Drawing for the job (mm, zero at the part's lowest x, y, z). A direction names the side the tool comes from. Round coordinates to 2 decimals unless told otherwise and drop trailing zeros. Loops run counter-clockwise (first coordinate to the right, second up) from the corner with the lowest first, then second, coordinate; pieces in that order, holes last. Notation, with made-up numbers: M 34,47.5 L 54,47.5 A21 ccw 54,75.5 Z; hole C 89,32.5 d1. An arc over 180 degrees is marked long. Answer in a Markdown table with one row per item.
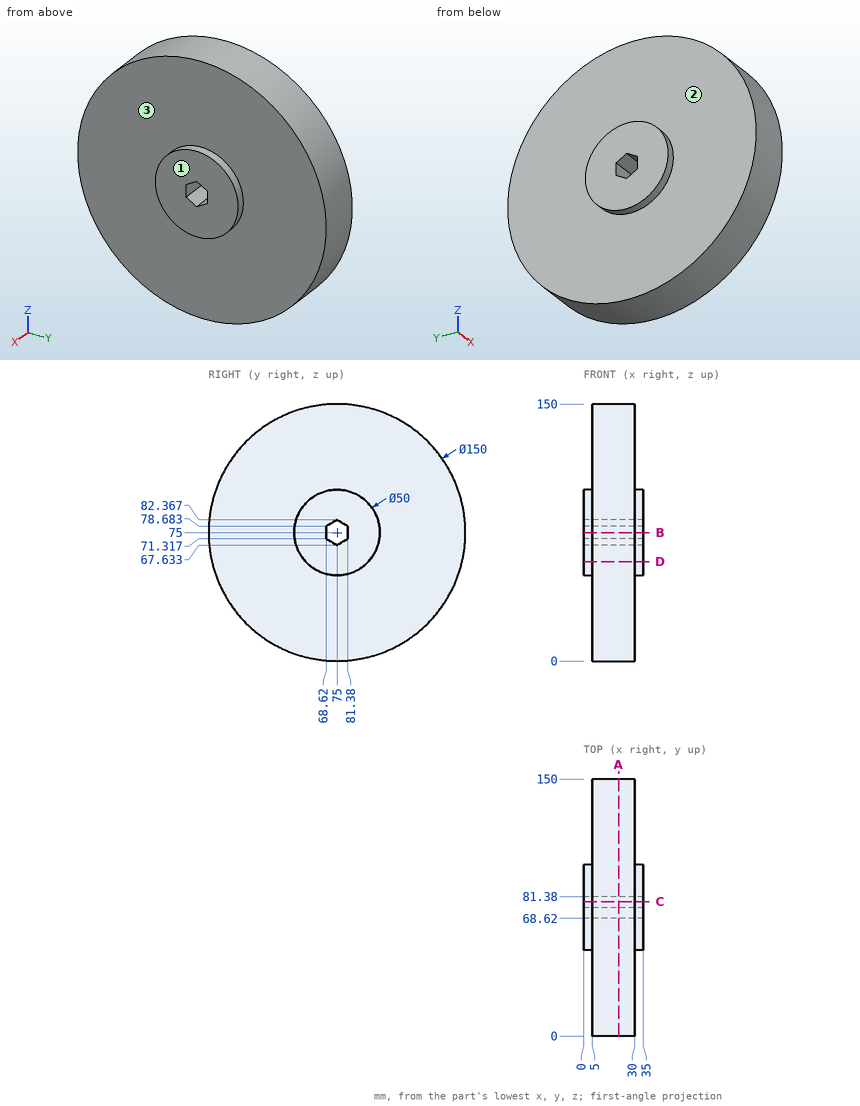
1. Saw through at C-C (y = 78.5). Write the cut outline in (x, z).
Verdict:
| item | result |
|---|---|
| outline | M 0,50.25 L 5,50.25 L 5,0.08 L 30,0.08 L 30,50.25 L 35,50.25 L 35,69.65 L 0,69.65 Z; M 0,80.35 L 35,80.35 L 35,99.75 L 30,99.75 L 30,149.92 L 5,149.92 L 5,99.75 L 0,99.75 Z |
2. Saw through at B-B (z = 75). Write the cut outline in (x, y), and give its area (3 significant figures).
Verdict:
| item | result |
|---|---|
| outline | M 0,50 L 5,50 L 5,0 L 30,0 L 30,50 L 35,50 L 35,68.62 L 0,68.62 Z; M 0,81.38 L 35,81.38 L 35,100 L 30,100 L 30,150 L 5,150 L 5,100 L 0,100 Z |
| area | 3,800 mm² |
3. Saw through at A-A (x = 20.5). Write the cut outline in (y, z), and give its area (3 significant figures).
Verdict:
| item | result |
|---|---|
| outline | C 75,75 d150; hole M 68.62,71.32 L 75,67.63 L 81.38,71.32 L 81.38,78.68 L 75,82.37 L 68.62,78.68 Z |
| area | 17,500 mm² |
4. Pin check, flat tips, straight feed: pin 1 (12 mm diameter, centred on x = 9.5, z = 48.5, fed in from +Y); pin 2 (1.5 mm diameter, centred on y = 39.5, z = 66.5, fed in from +X); pin 3 (10 mm diameter, centred on x = 6.5, y = 110, fed in from -Z). Stop position of each tip, or through.
Verdict:
| item | result |
|---|---|
| pin 1 | stops at y = 147.14 |
| pin 2 | stops at x = 30 |
| pin 3 | stops at z = 6.26 |
5. Saw through at D-D (z = 58). Write the cut outline in (x, y), and give its area (3 significant figures).
Verdict:
| item | result |
|---|---|
| outline | M 0,56.67 L 5,56.67 L 5,1.95 L 30,1.95 L 30,56.67 L 35,56.67 L 35,93.33 L 30,93.33 L 30,148.05 L 5,148.05 L 5,93.33 L 0,93.33 Z |
| area | 4,020 mm² |
6. Tool access for the marked faces 1, 2 and 3: list every direction of +Z, -Z, +X, -X, +Y, -Y with a clear straight run to the whole face (end or side of a thin tool).
Verdict:
| item | result |
|---|---|
| face 1 | +Z, -Z, +X, +Y, -Y |
| face 2 | -X |
| face 3 | +X |
7. Wall check: probe 1 along X at (y, z) = (111, 76); probe 2 along Y at (x, z) = (24.5, 76.5) (1 decimal); probe 3 along Y at (x, z) = (29, 15). Give the ranges that are in metal, low to high.
Verdict:
| item | result |
|---|---|
| probe 1 | x = 5 to 30 |
| probe 2 | y = 0 to 68.6, 81.4 to 150 |
| probe 3 | y = 30 to 120 |
